Design review of the part built by this model. Coordinates are the model's own, in mm. A direction names the side the tool comes from. Coordinates: 2 decimals unless noted, no trailing zeros. Write each loop counter-clockwise with the first axis right and the second up, starting at its lowest first coordinate (ties: lowest second). Pieces come first, ordered by that corner, then holes.
Q1. For pin 1 Ø0.9 at (y, z) = (-71, 118.5) entering from -X; pin 2 Ø0.6 at (y, z) = (71.5, 118) entering from -X; pin 3 Ø0.8 at (y, z) = (77, 119) entering from +X, all flat-tipped, find the tip position at first contact; note any pin that passes through.
Q2. The part is to be moulded in two halves that separate along Z. For faces 4 (the flat face through (-18.4, 78.4, 200)), 5 (the flat face through (-18.4, 78.4, 0)), 6 (the cylindrical face through (29.9, 74.8, 105.5)), say which applies: released by +Z, released by -Z, zero draft, split by the parting line, or undercut.
Q3. Take a section at D-D, the plane x = 30. Write out the cut boundary in (y, z), plus the area to 3 significant figures.
Q4. Take a section at B-B, the plane z = 68.5. Write out the cut boundary in (x, y).
Q5. For L1, parallel to Y at x = 0, z = 140; L2, parallel to Z at x = 121, y = 5; L3, parallel to X at y = -50, z = 99.5, list the stretches that pass through material, from the lowest coordinate up.
Q6. For faces 1 (the flat face through (77.058, -5.232, 107.873)), 2 (the cylindrical face through (29.9, -74.5, 105.5)), 3 (the cylindrical face through (80, 0, 115)), list the 3-axis set-ups (+Z, -Z, +X, -X, +Y, -Y) from which the entire face can be reached by the end or side of a thin tool; tool diameter is ignored.
Q7. Take a section at A-A, the plane x = -61. Write out the cut boundary in (y, z).
Q8. Take a section at C-C, the plane y = -16. Write out the cut boundary in (x, z).
from build123d import *

# Parameters (mm, degrees)
F0_R     = 81
F0_R_2   = 80
F1_DEPTH = 200
F3_DEPTH = 150
F6_R     = 1


with BuildPart() as f1:
    # F0 (on Top) → F1 (new body)
    with BuildSketch(Plane.XY):
        Circle(F0_R)
        Circle(F0_R_2, mode=Mode.SUBTRACT)
    extrude(amount=F1_DEPTH)

    # F2 (on Front) → F3 (cut, symmetric)
    with BuildSketch(Plane.XZ):
        with BuildLine():
            Line((37.5, 113), (37.5, 125))
            ThreePointArc((37.5, 125), (30, 132.5), (22.5, 125))
            Line((22.5, 125), (22.5, 113))
            ThreePointArc((22.5, 113), (30, 105.5), (37.5, 113))
        make_face()
    extrude(amount=F3_DEPTH, both=True, mode=Mode.SUBTRACT)

    # F4 (on Front) → F5 (revolve)
    with BuildSketch(Plane.XZ):
        Polygon((227.8234839022, 99.0889975246), (80.1023209503, 125.1362241746), (79.9286727727, 124.1514164216), (227.6498357245, 98.1041897716), align=None)
    revolve(axis=Axis((158.0200701243, 0, 101.2429566003), (0.984807753, 0, -0.1736481777)))

    # F6
    f6_edges = [f1.edges().sort_by_distance(p)[0] for p in [
        (80.380378, -9.99974, 114.85969),
        (80.380378, 9.99974, 114.85969),
    ]]
    fillet(f6_edges, radius=F6_R)


solid = f1.part
Responses:
1. pin 1: stops at x = -39.8
1. pin 2: stops at x = -38.62
1. pin 3: stops at x = 22.5
2. face 4: released by +Z
2. face 5: released by -Z
2. face 6: undercut
3. outline: (-75.24, 0) - (-74.16, 0) - (-74.16, 105.5) - (-75.24, 105.5) - close; (-75.24, 132.5) - (-74.16, 132.5) - (-74.16, 200) - (-75.24, 200) - close; (74.16, 0) - (75.24, 0) - (75.24, 105.5) - (74.16, 105.5) - close; (74.16, 132.5) - (75.24, 132.5) - (75.24, 200) - (74.16, 200) - close
3. area: 373 mm2
4. outline: circle Ø162 at (0, 0); hole circle Ø160 at (0, 0)
5. L1: y = -81 to -80, 80 to 81
5. L2: z = 98.98 to 100.17, 115.37 to 116.56
5. L3: x = -63.73 to -62.45, 62.45 to 63.73
6. face 1: +Z
6. face 2: +Y, -Y
6. face 3: none
7. outline: (-53.29, 0) - (-51.76, 0) - (-51.76, 200) - (-53.29, 200) - close; (51.76, 0) - (53.29, 0) - (53.29, 200) - (51.76, 200) - close
8. outline: (-79.4, 0) - (-78.38, 0) - (-78.38, 200) - (-79.4, 200) - close; (78.38, 0) - (79.4, 0) - (79.4, 200) - (78.38, 200) - close
